Design review of the part built by this model. Coordinates are the model's own, in mm. A direction names the side the tool comes from. Round coordinates to 2 decimals unless told otherwise and drop trailing zeros. Loops run counter-clockwise (first coordinate to the right, second up) from the corner with the lowest first, then second, coordinate; pieces in that order, holes last. Notation, with made-up numbers: M -36,45.25 L 7,45.25 A9 cw 7,59.25 Z; hole C -1.5,84 d10. An arc over 180 degrees is marked long. One line per item, written item: value. Start each with the question number.
Item 1: For faces 1 (the flat face through (38, 0.005, 25)), 2 (the flat face through (0, 20.005, 25)), 3 (the cylindrical face through (0.4, 25.04, 89.44)), list the 3-axis set-ups (+Z, -Z, +X, -X, +Y, -Y) from which the entire face can be reached by the end or side of a thin tool; tool diameter is ignored.
Item 2: Mouldability with a two-part tool opening along X and no side actions: class faces 4 (the cylindrical face through (0.132, 10.002, 49.646)), 5 (the flat face through (51, 20, 150)), 6 (the flat face through (-25.088, -8, 30)) as released by +X, released by -X, zero draft, split by the parting line, or undercut.
Item 3: We need section C-C (z = 3.5). Write out the cut boundary in (x, y).
Item 4: We need section D-D (x = -4). Write out the cut boundary in (y, z), then the cut area to 3 significant figures.
Item 5: For line 1 along Y through (x, z) = (51, 148.05); line 2 along Y through (x, z) = (15.25, 25); line 3 along Z through (x, y) = (40.5, 18.5), list the stretches that pass through material, from the lowest coordinate up.
Item 6: We need section B-B (x = 22.5). Write out the cut boundary in (y, z).
Item 7: Clearance check with flat-ended pins moving along their axes: pin 1 (2.5 mm diameter, centred on x = -51.5, y = 20.5, fed in from +Z); pin 2 (10 mm diameter, centred on x = -23, y = 5.5, fed in from +Z); pin 3 (1 mm diameter, centred on x = -19.5, z = 24.5, fed in from +Y). State where each tip first meets the part, or that it passes through.
Item 8: We need section A-A (z = 27.5). Write out the cut boundary in (x, y).
from build123d import *

# Parameters (mm, degrees)
BOSS_EXTRUDE1_DEPTH      = 50
SKETCH4_R                = 5
CUT_EXTRUDE1_DEPTH       = 116.323487875
FILLET2_R                = 20
SKETCH6_R                = 20
BOSS_EXTRUDE4_DEPTH      = 100
BOSS_EXTRUDE5_START      = 30
SKETCH7_R                = 20
BOSS_EXTRUDE5_DEPTH      = 30
SKETCH8_R                = 9.954491404
BOSS_EXTRUDE8_DEPTH      = 80
CUT_EXTRUDE2_DEPTH       = 130.001408198
CUT_EXTRUDE2_DEPTH_BACK  = 130.001408198
SKETCH9_R                = 13.643836255
CUT_EXTRUDE3_DEPTH       = 2
BOSS_EXTRUDE9_START      = 148
BOSS_EXTRUDE9_OUTLINE_R  = 5
BOSS_EXTRUDE9_DEPTH      = 1
CHAMFER1_SIZE            = 2
SKETCH11_R               = 13.6
CUT_EXTRUDE4_DEPTH       = 2
BOSS_EXTRUDE10_START     = 148
BOSS_EXTRUDE10_OUTLINE_R = 5
BOSS_EXTRUDE10_DEPTH     = 2
FILLET5_R                = 4
FILLET6_R                = 3
CHAMFER3_SIZE            = 2


# Read off the part's stored shape, not the designer's step: Boss-Extrude9, Boss-Extrude10
# Some blends are built 0.0001 mm under size
with BuildPart() as part:
    # Sketch1 → Boss-Extrude1 (new body)
    with BuildSketch(Plane.XY):
        with BuildLine():
            Line((-25.087834251, -19.995458795), (-10.087834251, -19.995458795))
            Line((-10.087834251, -19.995458795), (-10.087834251, 0.004541205))
            Line((-10.087834251, 0.004541205), (9.912165749, 0.004541205))
            Line((9.912165749, 0.004541205), (9.912165749, -19.995458795))
            Line((9.912165749, -19.995458795), (24.912165749, -19.995458795))
            Line((24.912165749, -19.995458795), (24.912165749, 0.004541205))
            Line((24.912165749, 0.004541205), (51, 0.004541205))
            ThreePointArc((51, 0.004541205), (65.142135624, 34.146676829), (31, 20.004541205))
            Line((31, 20.004541205), (-31, 20.004541205))
            ThreePointArc((-31, 20.004541205), (-65.142135624, 34.146676829), (-51, 0.004541205))
            Line((-51, 0.004541205), (-25.087834251, 0.004541205))
            Line((-25.087834251, 0.004541205), (-25.087834251, -19.995458795))
        make_face()
    extrude(amount=BOSS_EXTRUDE1_DEPTH)

    # Sketch4 → Cut-Extrude1 (cut, through all)
    with BuildSketch(Plane(origin=(24.912165749, 0, 0), x_dir=(0, 0, -1), z_dir=(1, 0, 0))):
        with Locations((-25, -9.995458795)):
            Circle(SKETCH4_R)
    extrude(amount=-CUT_EXTRUDE1_DEPTH, mode=Mode.SUBTRACT)

    # Fillet2
    fillet2_edges = [part.edges().sort_by_distance(p)[0] for p in [
        (-17.587834251, -19.995458795, 50),
        (-17.587834251, -19.995458795, 0),
        (17.412165749, -19.995458795, 0),
        (17.412165749, -19.995458795, 50),
    ]]
    fillet(fillet2_edges, radius=FILLET2_R)

    # Sketch6 → Boss-Extrude4 (add)
    with BuildSketch(Plane.XY.offset(50)):
        with Locations((-51, 20.004541205)):
            Circle(SKETCH6_R)
        with Locations(Location((51, 20.004541205, 0), (0, 0, 180))):
            Circle(SKETCH6_R)
    extrude(amount=BOSS_EXTRUDE4_DEPTH)

    # Sketch7 → Boss-Extrude5 (add)
    with BuildSketch(Plane(origin=(0, 0, 0), x_dir=(-1, 0, 0), z_dir=(0, 0, -1)).offset(BOSS_EXTRUDE5_START)):
        with Locations((-51, 20.004541205)):
            Circle(SKETCH7_R)
        with Locations((51, 20.004541205)):
            Circle(SKETCH7_R)
    extrude(amount=-BOSS_EXTRUDE5_DEPTH)

    # Sketch8 → Boss-Extrude8 (add)
    with BuildSketch(Plane.XY.offset(50)):
        with Locations(Location((0, 15.094063168, 0), (0, 0, 150.442767445))):
            Circle(SKETCH8_R)
    extrude(amount=BOSS_EXTRUDE8_DEPTH)

    # Sketch5 → Cut-Extrude2 (cut, two sides: drawn at the far end of the back side and taken through both)
    with BuildSketch(Plane.XY.offset(50).offset(-CUT_EXTRUDE2_DEPTH_BACK)):
        with BuildLine():
            Line((-10.087834251, 0.004541205), (9.912165749, 0.004541205))
            ThreePointArc((9.912165749, 0.004541205), (-0.087834251, 10.004541205), (-10.087834251, 0.004541205))
        make_face()
    extrude(amount=CUT_EXTRUDE2_DEPTH + CUT_EXTRUDE2_DEPTH_BACK, mode=Mode.SUBTRACT)

    # Sketch9 → Cut-Extrude3 (cut)
    with BuildSketch(Plane.XY.offset(150)):
        with Locations((-51, 20.004541205)):
            Circle(SKETCH9_R)
    extrude(amount=-CUT_EXTRUDE3_DEPTH, mode=Mode.SUBTRACT)

    # Boss-Extrude9 outline → Boss-Extrude9 (add)
    with BuildSketch(Plane.XY.offset(BOSS_EXTRUDE9_START)):
        with Locations((-51, 20.004541205)):
            Circle(BOSS_EXTRUDE9_OUTLINE_R)
    extrude(amount=BOSS_EXTRUDE9_DEPTH)

    # Chamfer1
    chamfer1_edges = [part.edges().sort_by_distance(p)[0] for p in [
        (-64.643836255, 20.004541205, 150),
    ]]
    chamfer(chamfer1_edges, length=CHAMFER1_SIZE - 0.0001)  # a hair under: the kernel refuses the full size

    # Sketch11 → Cut-Extrude4 (cut)
    with BuildSketch(Plane.XY.offset(150)):
        with Locations((51, 20.004541205)):
            Circle(SKETCH11_R)
    extrude(amount=-CUT_EXTRUDE4_DEPTH, mode=Mode.SUBTRACT)

    # Boss-Extrude10 outline → Boss-Extrude10 (add)
    with BuildSketch(Plane.XY.offset(BOSS_EXTRUDE10_START)):
        with Locations((51, 20.004541205)):
            Circle(BOSS_EXTRUDE10_OUTLINE_R)
    extrude(amount=BOSS_EXTRUDE10_DEPTH)

    # Fillet5
    # the kernel refuses this fillet: 4 mm, written as the material it takes off along each edge
    with BuildSketch(Plane(origin=(-51, 20.004541205, 149), x_dir=(1, 0, 0), z_dir=(0, -1, 0))) as fillet5_piece_1:
        with BuildLine():
            CenterArc((2.354248689, -4), FILLET5_R, 48.590377891, 41.409622109)
            Line((2.354248689, 0), (2.354248689, 0.08))
            Line((2.354248689, 0.08), (5, 0.08))
            Line((5, 0.08), (5.08, 0))
            ThreePointArc((5.08, 0), (5.08, -0.5), (5.052915026, -0.94))
            Line((5.052915026, -0.94), (5, -1))
        make_face()
    revolve(axis=Axis((-51, 20.004541205, 149), (0, 0, 1)), mode=Mode.SUBTRACT)

    # Fillet6
    # the kernel refuses this fillet: 3 mm, written as the material it takes off along each edge
    with BuildSketch(Plane(origin=(51, 20.004541205, 150), x_dir=(1, 0, 0), z_dir=(0, -1, 0))) as fillet6_piece_1:
        with BuildLine():
            CenterArc((2.171572875, -3), FILLET6_R, 19.471220634, 70.528779366)
            Line((2.171572875, 0), (2.171572875, 0.06))
            Line((2.171572875, 0.06), (5, 0.06))
            Line((5, 0.06), (5.06, 0))
            ThreePointArc((5.06, 0), (5.06, -1), (5.056568542, -1.98))
            Line((5.056568542, -1.98), (5, -2))
        make_face()
    revolve(axis=Axis((51, 20.004541205, 150), (0, 0, 1)), mode=Mode.SUBTRACT)

    # Chamfer3
    chamfer3_edges = [part.edges().sort_by_distance(p)[0] for p in [
        (37.4, 20.004541205, 150),
    ]]
    chamfer(chamfer3_edges, length=CHAMFER3_SIZE - 0.0001)  # a hair under: the kernel refuses the full size


solid = part.part
A:
1. face 1: +Z, -Z, +X, -Y
1. face 2: -Z, +Y
1. face 3: +Z
2. face 4: undercut
2. face 5: zero draft
2. face 6: released by -X
3. outline: M -51,0 L -25.09,0 L -25.09,-11.3 L -10.09,-11.3 L -10.09,0 A10 cw 9.91,0 L 9.91,-11.3 L 24.91,-11.3 L 24.91,0 L 51,0 A20 ccw long 31,20 L -31,20 A20 ccw long Z
4. outline: M 9.21,0 L 20,0 L 20,50 L 24.21,50 L 24.21,130 L 9.21,130 Z
4. area: 1,740 mm2
5. line 1: 0 to 6.35, 15.02 to 24.99, 33.65 to 40
5. line 2: -20 to -15, -5 to 20
5. line 3: -30 to 148
6. outline: M -20,20 A20 ccw 0,0 L 20,0 L 20,50 L 0,50 A20 ccw -20,30 Z; hole C -10,25 d10
7. pin 1: z = 149
7. pin 2: z = 50
7. pin 3: y = 20
8. outline: M -51,0 L -25.09,0 L -25.09,-5.67 L -10.09,-5.67 L -10.09,0 A10 cw 9.91,0 L 9.91,-5.67 L 24.91,-5.67 L 24.91,0 L 51,0 A20 ccw long 31,20 L -31,20 A20 ccw long Z; M -25.09,-20 L -10.09,-20 L -10.09,-14.33 L -25.09,-14.33 Z; M 9.91,-20 L 24.91,-20 L 24.91,-14.33 L 9.91,-14.33 Z
